Design review of the part built by this model. Coordinates are the model's own, in mm. A direction names the side the tool comes from. Give positions to 0.01 mm unless a question says otherwise; leave off trailing zeros. Write each loop counter-clockwise with the first axis right and the second up, starting at its lowest first coordinate (ties: lowest second). Pieces come first, ordered by that corner, then holes. Notation, with made-up numbers: M 57.25,22.25 L 75.25,22.25 A30 cw 75.25,50.25 Z; hole C -28,19 d6. An arc over 180 degrees is marked long. Use a Markdown table: item, result. Add a question column.
```python
from build123d import *

# Parameters (mm, degrees)
SKETCH1_W           = 304.8
SKETCH1_H           = 304.8
SKETCH1_W_2         = 254
SKETCH1_H_2         = 254
BOSS_EXTRUDE1_DEPTH = 6.35
FILLET1_R           = 76.2
FILLET2_R           = 12.7
SKETCH4_R           = 1.7653


with BuildPart() as part:
    # Sketch1 → Boss-Extrude1 (new body)
    with BuildSketch(Plane(origin=(0, 0, 0), x_dir=(1, 0, 0), z_dir=(0, 1, 0))):
        Rectangle(SKETCH1_W, SKETCH1_H)
        Rectangle(SKETCH1_W_2, SKETCH1_H_2, mode=Mode.SUBTRACT)
    extrude(amount=BOSS_EXTRUDE1_DEPTH)

    # Fillet1
    fillet1_edges = [part.edges().sort_by_distance(p)[0] for p in [
        (-127, 3.175, -127),
        (-127, 3.175, 127),
        (127, 3.175, 127),
        (127, 3.175, -127),
    ]]
    fillet(fillet1_edges, radius=FILLET1_R)

    # Fillet2
    fillet2_edges = [part.edges().sort_by_distance(p)[0] for p in [
        (152.4, 3.175, 152.4),
        (-152.4, 3.175, 152.4),
        (-152.4, 3.175, -152.4),
        (152.4, 3.175, -152.4),
    ]]
    fillet(fillet2_edges, radius=FILLET2_R)

    # Cut-Sweep1: sweep along a path in Sketch3
    with BuildLine(Plane(origin=(0, 6.35, 0), x_dir=(1, 0, 0), z_dir=(0, 1, 0))) as cut_sweep1_path:
        Line((114.3, -133.35), (-114.3, -133.35))
        ThreePointArc((-114.3, -133.35), (-127.770384182, -127.770384182), (-133.35, -114.3))
        Line((-133.35, -114.3), (-133.35, 114.3))
        ThreePointArc((-133.35, 114.3), (-127.770384182, 127.770384182), (-114.3, 133.35))
        Line((-114.3, 133.35), (114.3, 133.35))
        ThreePointArc((114.3, 133.35), (127.770384182, 127.770384182), (133.35, 114.3))
        Line((133.35, 114.3), (133.35, -114.3))
        ThreePointArc((133.35, -114.3), (127.770384182, -127.770384182), (114.3, -133.35))
    # Sketch4 → Cut-Sweep1 (sweep, cut)
    with BuildSketch(Plane(origin=(0, 0, 0), x_dir=(0, 0, -1), z_dir=(1, 0, 0))):
        with Locations((133.35, 6.35)):
            Circle(SKETCH4_R)
    sweep(path=cut_sweep1_path.line, mode=Mode.SUBTRACT)


solid = part.part
```
(1) Machinability: for faces 5 (the cylindrical face through (148.58, 3.22, 148.78)), 6 (the cylindrical face through (-104.086, 3.219, 105.271)), which of the approach directions +Z, -Z, +X, -X, +Y, -Y give a long, thin tool a straight path to every point of the face, cutting with its end or side? Answer none if there is none.
(2) Add section B-B on x = 24. Give the boundary of the cut face in (y, z).
(3) Add section C-C on y = 2.75. Give the boundary of the cut face in (x, z), then the cut area to 3 significant figures.
(4) Add section A-A on z = 32. Give the boundary of the cut face in (x, y), then the cut area to 3 significant figures.
(5) Wall thickness on L1, parallel to X at y = 0.5, z = -6.5; L2, parallel to Z at x = -80, y = 5.5: over which ranges is each line inside the solid? List them lowest first.
(6) The part is to be moulded in two halves that separate along X. For faces 1 (the cylindrical face through (148.58, 3.22, -148.78)), 2 (the cylindrical face through (104.086, 3.219, 105.271)), 3 (the flat face through (-136, 6.35, -23)), 4 (the cylindrical face through (-148.78, 3.22, -148.58)), say which applies: released by +X, released by -X, zero draft, split by the parting line, or undercut.
From the geometry:
| question | item | result |
|---|---|---|
| 1 | face 5 | +Z, +X, +Y, -Y |
| 1 | face 6 | +Y, -Y |
| 2 | outline | M 0,-152.4 L 6.35,-152.4 L 6.35,-135.12 A1.77 cw 6.35,-131.58 L 6.35,-127 L 0,-127 Z; M 0,127 L 6.35,127 L 6.35,131.58 A1.77 cw 6.35,135.12 L 6.35,152.4 L 0,152.4 Z |
| 3 | outline | M -152.4,-139.7 A12.7 ccw -139.7,-152.4 L 139.7,-152.4 A12.7 ccw 152.4,-139.7 L 152.4,139.7 A12.7 ccw 139.7,152.4 L -139.7,152.4 A12.7 ccw -152.4,139.7 Z; hole M -127,-50.8 A76.2 ccw -50.8,-127 L 50.8,-127 A76.2 ccw 127,-50.8 L 127,50.8 A76.2 ccw 50.8,127 L -50.8,127 A76.2 ccw -127,50.8 Z |
| 3 | area | 33,200 mm^2 |
| 4 | outline | M -152.4,0 L -127,0 L -127,6.35 L -131.58,6.35 A1.77 cw -135.12,6.35 L -152.4,6.35 Z; M 127,0 L 152.4,0 L 152.4,6.35 L 135.12,6.35 A1.77 cw 131.58,6.35 L 127,6.35 Z |
| 4 | area | 313 mm^2 |
| 5 | L1 | x = -152.4 to -127, 127 to 152.4 |
| 5 | L2 | z = -152.4 to -134.9, -131.8 to -121.18, 121.18 to 131.8, 134.9 to 152.4 |
| 6 | face 1 | released by +X |
| 6 | face 2 | undercut |
| 6 | face 3 | zero draft |
| 6 | face 4 | released by -X |
